The model under review builds one solid part; all positions refer to its coordinate system, in mm. A direction names the side the tool comes from. Round coordinates to 2 decimals unless told otherwise and drop trailing zeros. Write each loop counter-clockwise with the first axis right and the second up, starting at its lowest first coordinate (ties: lowest second). Pieces come first, ordered by that corner, then holes. Notation, with made-up numbers: M 4.5,26 L 54.5,26 A12 cw 54.5,47 Z; hole C -21.75,34 d6. An arc over 180 degrees is marked long. Write item = value, one per line. Start each with the question number.
Item 1: Tool access review of faces 1 (the flat face through (1.3, 79, 11)), 2 (the cylindrical face through (7.1, 142.6, 0.7)), 3 (the flat face through (20, 16, 5)): name each direction out of +Z, -Z, +X, -X, +Y, -Y from which nothing blocks a thin tool from reaching the whole face with its end or side.
Item 2: The part is to be moulded in two halves that separate along X. For faces 4 (the flat face through (101, 143, 1.5)), 5 (the flat face through (53, 160, 3)), 6 (the flat face through (108, 79, 10)), say which applies: +X half, -X half, draft (parallel to the pull), parting line (faces both ways), or undercut.
Item 3: To check wall thickness, follow line 1 along Y through (x, z) = (100.35, 3.25); line 2 along X through (y, z) = (21.95, 0.85); line 3 along Y through (x, z) = (7.65, 0.4). State the ranges of each line that lie inside material, in increasing order.
Item 4: Take a section at B-B, the plane x = 100.35. Give the number of separate pieces and of enclosed holes in the cut face, plus the area to 3 significant figures.
Item 5: For pin 1 Ø8 at (x, y) = (51.5, 135.5) entering from +Z; pin 2 Ø1 at (x, y) = (34.5, 139) entering from -Z; pin 3 Ø7.5 at (x, y) = (8.5, 21.5) entering from +Z; pin 4 Ø0.6 at (y, z) = (16, 6.5) entering from -X, all flat-tipped, find the tip position at first contact; note any pin that passes through.
Item 6: Take a section at D-D, the plane y = 41. Give the boundary of the cut face in (x, z), plus the area to 3 significant figures.
Item 7: Take a section at A-A, the plane x = 69.5. Give the boundary of the cut face in (y, z), plus the area to 3 significant figures.
from build123d import *

# Parameters (mm, degrees)
BOX015_W          = 28
BOX015_H          = 8.5
BOX015_DEPTH      = 10
BOX016_W          = 28
BOX016_H          = 8.5
BOX016_DEPTH      = 10
BOX014_W          = 50
BOX014_H          = 12
BOX014_DEPTH      = 3
BOX013_W          = 52.6
BOX013_H          = 14.6
BOX013_DEPTH      = 3
CYLINDER006_R     = 2.6
CYLINDER006_DEPTH = 1.5
CYLINDER005_R     = 1.7
CYLINDER005_DEPTH = 5
CYLINDER_R        = 3.5
CYLINDER_DEPTH    = 5
CYLINDER001_R     = 3.5
CYLINDER001_DEPTH = 5
CYLINDER002_R     = 3.5
CYLINDER002_DEPTH = 5
CYLINDER003_R     = 3.5
CYLINDER003_DEPTH = 5
BOX012_W          = 48
BOX012_H          = 1.3
BOX012_DEPTH      = 16
BOX008_W          = 60
BOX008_H          = 13
BOX008_DEPTH      = 1.6
BOX002_W          = 80
BOX002_H          = 17
BOX002_DEPTH      = 13
BOX001_W          = 105.4
BOX001_H          = 157.4
BOX001_DEPTH      = 19
BOX_W             = 108
BOX_H             = 160
BOX_DEPTH         = 21
BOX007_W          = 55
BOX007_H          = 4.5
BOX007_DEPTH      = 2
BOX006_W          = 82.6
BOX006_H          = 2
BOX006_DEPTH      = 7.4
BOX005_W          = 80
BOX005_H          = 14
BOX005_DEPTH      = 8
BOX004_W          = 80
BOX004_H          = 17
BOX004_DEPTH      = 5
BOX003_W          = 82.6
BOX003_H          = 18.3
BOX003_DEPTH      = 14.3
BOX009_W          = 62.6
BOX009_H          = 15.6
BOX009_DEPTH      = 1.7


with BuildPart() as board_pusher_left:
    # Box015 → Box015 (new body)
    with BuildSketch(Plane(origin=(1.3, 150.2, 2), x_dir=(1, 0, 0), z_dir=(0, 0, 1))):
        with Locations((14, 4.25)):
            Rectangle(BOX015_W, BOX015_H)
    extrude(amount=BOX015_DEPTH)


with BuildPart() as board_pusher_right:
    # Box016 → Box016 (new body)
    with BuildSketch(Plane(origin=(78.7, 150.2, 2), x_dir=(1, 0, 0), z_dir=(0, 0, 1))):
        with Locations((14, 4.25)):
            Rectangle(BOX016_W, BOX016_H)
    extrude(amount=BOX016_DEPTH)


with BuildPart() as board_support_inner:
    # Box014 → Box014 (new body)
    with BuildSketch(Plane(origin=(29, 146.7, 2), x_dir=(1, 0, 0), z_dir=(0, 0, 1))):
        with Locations((25, 6)):
            Rectangle(BOX014_W, BOX014_H)
    extrude(amount=BOX014_DEPTH)


with BuildPart() as board_support:
    # Box013 → Box013 (new body)
    with BuildSketch(Plane(origin=(27.7, 145.4, 2), x_dir=(1, 0, 0), z_dir=(0, 0, 1))):
        with Locations((26.3, 7.3)):
            Rectangle(BOX013_W, BOX013_H)
    extrude(amount=BOX013_DEPTH)

    # Cut008: cut Board support inner
    add(board_support_inner.part, mode=Mode.SUBTRACT)


with BuildPart() as bottom_hole:
    # Cylinder006 → Cylinder006 (new body)
    with BuildSketch(Plane(origin=(7.65, 145.14, 0), x_dir=(1, 0, 0), z_dir=(0, 0, 1))):
        Circle(CYLINDER006_R)
    extrude(amount=CYLINDER006_DEPTH)


with BuildPart() as hole1:
    # Cylinder005 → Cylinder005 (new body)
    with BuildSketch(Plane(origin=(7.65, 145.14, 0), x_dir=(1, 0, 0), z_dir=(0, 0, 1))):
        Circle(CYLINDER005_R)
    extrude(amount=CYLINDER005_DEPTH)

    # Fusion003: union Bottom hole
    add(bottom_hole.part)


with BuildPart() as hole2:
    # Clone base: copy of Hole1
    add(hole1.part)


with BuildPart() as hole2_1:
    # Clone placement: moved
    add(hole2.part.moved(Location((92.7, 0, 0))))


with BuildPart() as hole3:
    # Clone001 base: copy of Hole2
    add(hole2_1.part)


with BuildPart() as hole3_1:
    # Clone001 placement: moved
    add(hole3.part.moved(Location((-92.7, -123.19, 0))))


with BuildPart() as hole4:
    # Clone002 base: copy of Hole3
    add(hole3_1.part)


with BuildPart() as hole4_1:
    # Clone002 placement: moved
    add(hole4.part.moved(Location((92.7, 0, 0))))


with BuildPart() as holes:
    # Fusion004 base: copy of Hole1
    add(hole1.part)

    # Fusion004: union Hole4, Hole3, Hole2
    add(hole4_1.part)
    add(hole3_1.part)
    add(hole2_1.part)


with BuildPart() as cylinder:
    # Cylinder → Cylinder (new body)
    with BuildSketch(Plane(origin=(7.65, 145.14, 0), x_dir=(1, 0, 0), z_dir=(0, 0, 1))):
        Circle(CYLINDER_R)
    extrude(amount=CYLINDER_DEPTH)


with BuildPart() as cylinder001:
    # Cylinder001 → Cylinder001 (new body)
    with BuildSketch(Plane(origin=(100.35, 145.14, 0), x_dir=(1, 0, 0), z_dir=(0, 0, 1))):
        Circle(CYLINDER001_R)
    extrude(amount=CYLINDER001_DEPTH)


with BuildPart() as cylinder002:
    # Cylinder002 → Cylinder002 (new body)
    with BuildSketch(Plane(origin=(7.65, 21.95, 0), x_dir=(1, 0, 0), z_dir=(0, 0, 1))):
        Circle(CYLINDER002_R)
    extrude(amount=CYLINDER002_DEPTH)


with BuildPart() as cylinder003:
    # Cylinder003 → Cylinder003 (new body)
    with BuildSketch(Plane(origin=(100.35, 21.95, 0), x_dir=(1, 0, 0), z_dir=(0, 0, 1))):
        Circle(CYLINDER003_R)
    extrude(amount=CYLINDER003_DEPTH)


with BuildPart() as obj1:
    # Box012 → Box012 (new body)
    with BuildSketch(Plane(origin=(30, 158.7, 5), x_dir=(1, 0, 0), z_dir=(0, 0, 1))):
        with Locations((24, 0.65)):
            Rectangle(BOX012_W, BOX012_H)
    extrude(amount=BOX012_DEPTH)


with BuildPart() as bottom_cutout:
    # Box008 → Box008 (new body)
    with BuildSketch(Plane(origin=(24, 131.1, 0), x_dir=(1, 0, 0), z_dir=(0, 0, 1))):
        with Locations((30, 6.5)):
            Rectangle(BOX008_W, BOX008_H)
    extrude(amount=BOX008_DEPTH)


with BuildPart() as cube002:
    # Box002 → Box002 (new body)
    with BuildSketch(Plane(origin=(14, 0, 0), x_dir=(1, 0, 0), z_dir=(0, 0, 1))):
        with Locations((40, 8.5)):
            Rectangle(BOX002_W, BOX002_H)
    extrude(amount=BOX002_DEPTH)


with BuildPart() as cube001:
    # Box001 → Box001 (new body)
    with BuildSketch(Plane(origin=(1.3, 1.3, 2), x_dir=(1, 0, 0), z_dir=(0, 0, 1))):
        with Locations((52.7, 78.7)):
            Rectangle(BOX001_W, BOX001_H)
    extrude(amount=BOX001_DEPTH)


with BuildPart() as obj2:
    # Box → Box (new body)
    with BuildSketch(Plane.XY):
        with Locations((54, 80)):
            Rectangle(BOX_W, BOX_H)
    extrude(amount=BOX_DEPTH)

    # Cut: cut Cube001
    add(cube001.part, mode=Mode.SUBTRACT)

    # Cut001: cut Cube002
    add(cube002.part, mode=Mode.SUBTRACT)


with BuildPart() as board_carve:
    # Box007 → Box007 (new body)
    with BuildSketch(Plane(origin=(26.5, 14, 5), x_dir=(1, 0, 0), z_dir=(0, 0, 1))):
        with Locations((27.5, 2.25)):
            Rectangle(BOX007_W, BOX007_H)
    extrude(amount=BOX007_DEPTH)


with BuildPart() as obj3:
    # Box006 → Box006 (new body)
    with BuildSketch(Plane(origin=(12.7, 16.3, 6.9), x_dir=(1, 0, 0), z_dir=(0, 0, 1))):
        with Locations((41.3, 1)):
            Rectangle(BOX006_W, BOX006_H)
    extrude(amount=BOX006_DEPTH)


with BuildPart() as obj4:
    # Box005 → Box005 (new body)
    with BuildSketch(Plane(origin=(14, 0, 5), x_dir=(1, 0, 0), z_dir=(0, 0, 1))):
        with Locations((40, 7)):
            Rectangle(BOX005_W, BOX005_H)
    extrude(amount=BOX005_DEPTH)


with BuildPart() as obj5:
    # Box004 → Box004 (new body)
    with BuildSketch(Plane(origin=(14, 0, 0), x_dir=(1, 0, 0), z_dir=(0, 0, 1))):
        with Locations((40, 8.5)):
            Rectangle(BOX004_W, BOX004_H)
    extrude(amount=BOX004_DEPTH)


with BuildPart() as board_with_holes:
    # Box003 → Box003 (new body)
    with BuildSketch(Plane(origin=(12.7, 0, 0), x_dir=(1, 0, 0), z_dir=(0, 0, 1))):
        with Locations((41.3, 9.15)):
            Rectangle(BOX003_W, BOX003_H)
    extrude(amount=BOX003_DEPTH)

    # Cut002: cut obj5
    add(obj5.part, mode=Mode.SUBTRACT)

    # Cut003: cut obj4
    add(obj4.part, mode=Mode.SUBTRACT)

    # Cut004: cut obj3
    add(obj3.part, mode=Mode.SUBTRACT)

    # Cut005: cut Board carve
    add(board_carve.part, mode=Mode.SUBTRACT)

    # Fusion: union obj2
    add(obj2.part)

    # Cut006: cut Bottom cutout
    add(bottom_cutout.part, mode=Mode.SUBTRACT)

    # Cut007: cut obj1
    add(obj1.part, mode=Mode.SUBTRACT)

    # Fusion002: union Cylinder, Cylinder001, Cylinder002, Cylinder003
    add(cylinder.part)
    add(cylinder001.part)
    add(cylinder002.part)
    add(cylinder003.part)

    # Cut009: cut Holes
    add(holes.part, mode=Mode.SUBTRACT)


with BuildPart() as all_case_parts:
    # Box009 → Box009 (new body)
    with BuildSketch(Plane(origin=(22.7, 129.8, 1.6), x_dir=(1, 0, 0), z_dir=(0, 0, 1))):
        with Locations((31.3, 7.8)):
            Rectangle(BOX009_W, BOX009_H)
    extrude(amount=BOX009_DEPTH)

    # Fusion005: union Board pusher left, Board pusher right, Board Support, Board with holes
    add(board_pusher_left.part)
    add(board_pusher_right.part)
    add(board_support.part)
    add(board_with_holes.part)


solid = all_case_parts.part
Response values:
q1.face_1 = +Z
q1.face_2 = -Z
q1.face_3 = -Z, -Y
q2.face_4 = undercut
q2.face_5 = draft
q2.face_6 = +X half
q3.line_1 = 0 to 1.3, 18.45 to 20.25, 23.65 to 25.45, 141.64 to 143.44, 146.84 to 148.64, 150.2 to 160
q3.line_2 = 0 to 5.05, 10.25 to 97.75, 102.95 to 108
q3.line_3 = 0 to 19.35, 24.55 to 142.54, 147.74 to 160
q4.separate_pieces = 3
q4.enclosed_holes = 0
q4.area = 457 mm2
q5.pin_1 = 3.3
q5.pin_2 = 1.6
q5.pin_3 = 5
q5.pin_4 = 0
q6.outline = M 0,0 L 108,0 L 108,21 L 106.7,21 L 106.7,2 L 1.3,2 L 1.3,21 L 0,21 Z
q6.area = 265 mm2
q7.outline = M 0,13 L 14,13 L 14,7 L 16.3,7 L 16.3,14.3 L 1.3,14.3 L 1.3,21 L 0,21 Z; M 17,0 L 131.1,0 L 131.1,1.6 L 144.1,1.6 L 144.1,0 L 160,0 L 160,5 L 158.7,5 L 158.7,2 L 146.7,2 L 146.7,5 L 145.4,5 L 145.4,3.3 L 129.8,3.3 L 129.8,2 L 18.3,2 L 18.3,5 L 17,5 Z
q7.area = 341 mm2
